Part model, mm, in its own coordinate system. A direction names the side the tool comes from. Give positions to 0.01 mm unless a question says otherwise; leave off trailing zeros. Order: outer loops, then holes, each group sorted by start corner. A loop starts at its lowest first (then second) coordinate and runs counter-clockwise, first axis right, second up.
1. Probe line 1 (X direction, y = 5, z = 11.25); line 2 (X direction, y = 24, z = 17); line 3 (Y direction, x = -4, z = 17.75). List the from-to ranges inside material, lowest first.
2. Drop flat-ended pins along their axis: pin 1 Ø2.5 at (x, y) = (-34.98, -1.92) entering from +Z; pin 2 Ø2 at (y, z) = (3.5, 11) entering from +X; pin 3 Ø3 at (x, z) = (2.5, 16) entering from -Y; pin 4 Ø3 at (y, z) = (-2, 14) entering from +X. Give the stop position or say it passes through.
3. Mould opens along X. For faces 1 (the flat face through (-1.737, 40.062, 13.944)), 2 (the flat face through (-37.48, 36, 11)), 3 (the flat face through (-38, 21, 18)) say: +X half, -X half, draft (parallel to the pull), parting line (faces both ways), or undercut.
4. Slice it at D-D on z = 16.5. List the corners of the cut face in (x, y).
5. Slice it at B-B on y = 19. List the corners of the cut face in (x, z).
6. Slice it at C-C on x = -10. List the corners of the cut face in (y, z).
7. Which spindle directions (+Z, -Z, +X, -X, +Y, -Y) get a long thin tool onto all of the face, cutting with end or side? Do faces 4 (the flat face through (-21, 42.38, 11)), 5 (the flat face through (-3.93, -2, 14)), 6 (the flat face through (-21, 2.38, 15)). Say none if no direction does.
Autodesk Inventor part; units mm, degrees
ref_plane "Work Plane1" through (0, 0, 10) normal (0, 0, 1) x (1, 0, 0)
ref_plane "YZ Plane" through (0, 0, 0) normal (1, 0, 0) x (0, 1, 0)
ref_plane "XZ Plane" through (0, 0, 0) normal (0, 1, 0) x (-1, 0, 0)
ref_plane "Work Plane1" through (0, 0, 10) normal (0, 0, 1) x (1, 0, 0)
sketch "Sketch1" plane through (0, 0, 10) normal (0, 0, 1) x (1, 0, 0)
  line L0 (-4.0299, -0.3538) -> (-2.2322, 1.4439) construction
  arc A0 (-1.4439, 2.2322) -> (-2.2322, 1.4439) centre (-0.9299, 0.9299) ccw construction
  line L1 (-1.4439, 2.2322) -> (0.3538, 4.0299) construction
  line L2 (-37.8299, 42.2137) -> (-37.8299, 45.8299) construction
  line L3 (-37.8299, 45.8299) -> (-4.0299, 45.8299) construction
  line L4 (-4.0299, 45.8299) -> (-4.0299, 42.2137) construction
  line L5 (-4.0299, 4.0299) -> (0.3538, 4.0299)
  circle A1 centre (-20.9299, 20.9299) radius 17.5 construction
  line L6 (-20.9299, 58.9723) -> (17.1124, 20.9299) construction
  line L7 (17.1124, 20.9299) -> (-20.9299, -17.1124) construction
  line L8 (-20.9299, -17.1124) -> (-58.9723, 20.9299) construction
  line L9 (-58.9723, 20.9299) -> (-20.9299, 58.9723) construction
  line L10 (-20.9299, 58.9723) -> (-20.9299, -17.1124) construction
  line L11 (17.1124, 20.9299) -> (-58.9723, 20.9299) construction
  line L12 (-20.9299, 58.9723) -> (32.8701, 58.9723) construction
  line L13 (-43.2198, 43.4299) -> (1.7802, 43.4299) construction
  line L14 (1.7802, 43.4299) -> (1.7802, -1.5701) construction
  line L15 (1.7802, -1.5701) -> (-43.2198, -1.5701) construction
  line L16 (-43.2198, -1.5701) -> (-43.2198, 43.4299) construction
  line L17 (-43.2198, 5.1774) -> (-43.2198, 36.6824)
  line L18 (-43.2198, 36.6824) -> (-36.4723, 43.4299)
  line L19 (-36.4723, 43.4299) -> (-5.3876, 43.4299)
  line L20 (-5.3876, 43.4299) -> (1.7802, 36.2621)
  line L21 (1.7802, 36.2621) -> (1.7802, 5.5977)
  line L22 (1.7802, 5.5977) -> (-5.3876, -1.5701)
  line L23 (-5.3876, -1.5701) -> (-36.4723, -1.5701)
  line L24 (-36.4723, -1.5701) -> (-43.2198, 5.1774)
  line L25 (-4.0299, 42.2137) -> (-37.8299, 42.2137)
  line L26 (-4.0299, -0.3538) -> (-4.0299, 4.0299)
  line L27 (-43.2198, 43.4299) -> (-10.4667, 10.6769) construction
  line L28 (-8.5595, 8.5517) -> (1.7802, -1.5701) construction
  line L29 (1.7802, 43.4299) -> (-25.699, 15.9507) construction
  line L30 (-30.9728, 10.6769) -> (-43.2198, -1.5701) construction
  point P0 (-37.8299, 4.0299)
  dimension "d18" = 53.8
  dimension "d19" = 45
  dimension "d20" = 53.8
  dimension "d21" = 45
  dimension "d22" = 45
extrude "Extrusion1" add sketch "Sketch1" along normal blind 8
sketch "Sketch3" plane through (0, 0, 10) normal (0, 0, -1) x (-1, 0, 0)
  line L0 (37.8299, -0.4701) -> (37.8299, 4.0299) construction
  line L1 (4.0299, 4.0299) -> (4.0299, -0.4701) construction
  line L2 (37.8299, -0.4701) -> (37.8299, 1.1886) construction
  line L3 (4.0299, -3.9701) -> (4.0299, -0.3538) construction
  line L4 (45.8299, 4.0299) -> (42.2137, 4.0299) construction
  line L5 (-0.3538, 4.0299) -> (-3.9701, 4.0299) construction
  line L6 (-3.9701, 37.8299) -> (-0.3538, 37.8299) construction
  line L7 (4.0299, 42.2137) -> (4.0299, 45.8299) construction
  line L8 (37.8299, 45.8299) -> (37.8299, 42.2137) construction
  line L9 (42.2137, 37.8299) -> (45.8299, 37.8299) construction
  line L10 (37.8299, 37.7299) -> (45.8299, 37.7299)
  line L11 (45.8299, 37.7299) -> (45.8299, 4.1299)
  line L12 (45.8299, 4.1299) -> (37.8299, 4.1299)
  line L13 (37.8299, 4.1299) -> (37.8299, 37.7299)
  line L14 (37.7299, 4.0299) -> (4.1299, 4.0299)
  line L15 (4.1299, 4.0299) -> (4.1299, -3.9701)
  line L16 (4.1299, -3.9701) -> (37.7299, -3.9701)
  line L17 (37.7299, -3.9701) -> (37.7299, 4.0299)
  line L18 (4.0299, 4.1299) -> (-3.9701, 4.1299)
  line L19 (-3.9701, 4.1299) -> (-3.9701, 37.7299)
  line L20 (-3.9701, 37.7299) -> (4.0299, 37.7299)
  line L21 (4.0299, 37.7299) -> (4.0299, 4.1299)
  line L22 (4.1299, 37.8299) -> (37.7299, 37.8299)
  line L23 (37.7299, 37.8299) -> (37.7299, 45.8299)
  line L24 (37.7299, 45.8299) -> (4.1299, 45.8299)
  line L25 (4.1299, 45.8299) -> (4.1299, 37.8299)
  point P0 (0, 0)
  dimension "d23" = 0.1
  dimension "d24" = 0.1
  dimension "d25" = 0.1
  dimension "d26" = 0.1
  dimension "d27" = 0.1
extrude "Extrusion3" add sketch "Sketch3" against normal up to surface (8 mm away)
sketch "Skizze12" plane through (0, 0, 10) normal (0, 0, -1) x (-1, 0, 0)
  line L0 (-0.3124, 4.1299) -> (4.1299, -0.3124)
  line L1 (4.1299, -0.3124) -> (4.1299, -3.9701)
  line L2 (4.1299, -3.9701) -> (37.7299, -3.9701) construction
  line L3 (37.7299, -3.9701) -> (37.7299, -0.3124)
  line L4 (37.7299, -0.3124) -> (42.1723, 4.1299)
  line L5 (45.8299, 4.1299) -> (42.1723, 4.1299)
  line L6 (45.8299, 37.7299) -> (45.8299, 4.1299) construction
  line L7 (42.1723, 37.7299) -> (45.8299, 37.7299)
  line L8 (42.1723, 37.7299) -> (37.7299, 42.1723)
  line L9 (37.7299, 42.1723) -> (37.7299, 45.8299)
  line L10 (37.7299, 45.8299) -> (4.1299, 45.8299) construction
  line L11 (4.1299, 45.8299) -> (4.1299, 42.1723)
  line L12 (4.1299, 42.1723) -> (-0.3124, 37.7299)
  line L13 (-3.9701, 37.7299) -> (-0.3124, 37.7299)
  line L14 (-3.9701, 4.1299) -> (-3.9701, 37.7299) construction
  line L15 (-0.3124, 4.1299) -> (-3.9701, 4.1299)
  line L16 (37.9299, -4.1701) -> (3.9299, -4.1701) construction
  line L17 (3.9299, -4.1701) -> (3.9299, -0.3953)
  line L18 (3.9299, -0.3953) -> (-0.3953, 3.9299)
  line L19 (-0.3953, 3.9299) -> (-4.1701, 3.9299)
  line L20 (-4.1701, 3.9299) -> (-4.1701, 37.9299) construction
  line L21 (-4.1701, 37.9299) -> (-0.3953, 37.9299)
  line L22 (-0.3953, 37.9299) -> (3.9299, 42.2551)
  line L23 (3.9299, 42.2551) -> (3.9299, 46.0299)
  line L24 (3.9299, 46.0299) -> (37.9299, 46.0299) construction
  line L25 (37.9299, 46.0299) -> (37.9299, 42.2551)
  line L26 (37.9299, 42.2551) -> (42.2551, 37.9299)
  line L27 (42.2551, 37.9299) -> (46.0299, 37.9299)
  line L28 (46.0299, 37.9299) -> (46.0299, 3.9299) construction
  line L29 (46.0299, 3.9299) -> (42.2551, 3.9299)
  line L30 (42.2551, 3.9299) -> (37.9299, -0.3953)
  line L31 (37.9299, -0.3953) -> (37.9299, -4.1701)
  line L32 (-3.9701, 37.7299) -> (-3.9701, 37.9299)
  line L33 (37.7299, 45.8299) -> (4.1299, 45.8299)
  line L34 (4.1299, 45.8299) -> (3.9299, 45.8299)
  line L35 (37.7299, 45.8299) -> (37.9299, 45.8299)
  line L36 (45.8299, 37.7299) -> (45.8299, 37.9299)
  line L37 (45.8299, 4.1299) -> (45.8299, 3.9299)
  line L38 (37.7299, -3.9701) -> (37.9299, -3.9701)
  line L39 (4.1299, -3.9701) -> (3.9299, -3.9701)
  line L40 (-3.9701, 4.1299) -> (-3.9701, 3.9299)
  point P0 (0, 0)
  dimension "d65" = 0.2
extrude "IM_offset" add sketch "Skizze12" against normal up to surface (8 mm away)
sketch "Sketch15" plane through (0, 0, 10) normal (0, 0, -1) x (-1, 0, 0)
  line L0 (-3.9701, 3.9299) -> (-3.9701, 37.9299)
  line L1 (-0.3953, 3.9299) -> (-3.9701, 3.9299)
  line L2 (3.9299, -0.3953) -> (-0.3953, 3.9299)
  line L3 (3.9299, -3.9701) -> (3.9299, -0.3953)
  line L4 (3.9299, -3.9701) -> (37.9299, -3.9701)
  line L5 (37.9299, -0.3953) -> (37.9299, -3.9701)
  line L6 (42.2551, 3.9299) -> (37.9299, -0.3953)
  line L7 (45.8299, 3.9299) -> (42.2551, 3.9299)
  line L8 (45.8299, 3.9299) -> (45.8299, 37.9299)
  line L9 (45.8299, 37.9299) -> (42.2551, 37.9299)
  line L10 (42.2551, 37.9299) -> (37.9299, 42.2551)
  line L11 (37.9299, 42.2551) -> (37.9299, 45.8299)
  line L12 (37.9299, 45.8299) -> (3.9299, 45.8299)
  line L13 (3.9299, 45.8299) -> (3.9299, 42.2551)
  line L14 (3.9299, 42.2551) -> (-0.3953, 37.9299)
  line L15 (-0.3953, 37.9299) -> (-3.9701, 37.9299)
  line L16 (37.4799, 42.3799) -> (4.4799, 42.3799)
  line L17 (4.4799, 42.3799) -> (4.4799, -0.6201)
  line L18 (4.4799, -0.6201) -> (37.4799, -0.6201)
  line L19 (37.4799, -0.6201) -> (37.4799, 42.3799)
  line L20 (37.4799, 42.3799) -> (4.4799, -0.6201) construction
  line L21 (4.4799, 42.3799) -> (37.4799, -0.6201) construction
  circle A0 centre (20.9799, 20.8799) radius 16.97 construction
  point P0 (0, 0)
  dimension "d73" = 33
  dimension "d74" = 43
  dimension "d90" = 21.5
  dimension "d91" = 16.5
extrude "Extrusion13" cut sketch "Sketch15" against normal blind 2 contours L19 L18 L17 L16
sketch "Sketch16" plane through (0, 0, 12) normal (0, 0, -1) x (-1, 0, 0)
  line L0 (4.4799, 42.3799) -> (37.4799, 42.3799)
  line L1 (4.4799, -0.6201) -> (4.4799, 42.3799)
  line L2 (37.4799, -0.6201) -> (4.4799, -0.6201)
  line L3 (37.4799, 42.3799) -> (37.4799, -0.6201)
  line L4 (7.4799, 39.3799) -> (34.4799, 39.3799)
  line L5 (34.4799, 39.3799) -> (34.4799, 2.3799)
  line L6 (34.4799, 2.3799) -> (7.4799, 2.3799)
  line L7 (7.4799, 2.3799) -> (7.4799, 39.3799)
  dimension "d94" = 3
extrude "Extrusion14" cut sketch "Sketch16" against normal through all contours L4 L5 L6 L7
sketch "Sketch17" plane through (0, 0, 10) normal (0, 0, -1) x (-1, 0, 0)
  line L0 (37.4799, 42.3799) -> (37.4799, -0.6201)
  line L1 (4.4799, -0.6201) -> (4.4799, 42.3799)
  line L2 (38.7299, 28.3799) -> (3.2299, 28.3799)
  line L3 (3.2299, 28.3799) -> (3.2299, 13.3799)
  line L4 (3.2299, 13.3799) -> (38.7299, 13.3799)
  line L5 (38.7299, 13.3799) -> (38.7299, 28.3799)
  line L6 (38.7299, 28.3799) -> (3.2299, 13.3799) construction
  line L7 (3.2299, 28.3799) -> (38.7299, 13.3799) construction
  line L8 (4.4799, 42.3799) -> (37.4799, 42.3799)
  circle A0 centre (20.9799, 20.8799) radius 16.97 construction
  line L9 (37.4799, -0.6201) -> (4.4799, -0.6201)
  point P0 (0, 0)
  dimension "d81" = 35.5
  dimension "d82" = 15
  dimension "d92" = 0
  dimension "d93" = 0
hole "Hole1" at (-3.2299, 13.3799, 10) at (-3.2299, 28.3799, 10) at (-38.7299, 28.3799, 10) at (-38.7299, 13.3799, 10) direction (0, 0, 1) diameter 2.8 end through all
sketch "Sketch18" plane through (0, 0, 10) normal (0, 0, -1) x (-1, 0, 0)
  line L0 (45.3299, 43.7299) -> (45.3299, -1.9701)
  line L1 (37.9499, -0.2701) -> (37.9499, -3.9701)
  line L2 (4.0099, -3.9701) -> (4.0099, 0.1299)
  circle A0 centre (6.9799, -1.9201) radius 1.4
  circle A1 centre (34.9799, -1.9201) radius 1.4
  circle A2 centre (20.9799, 20.8799) radius 16.97 construction
  circle A3 centre (20.9799, 20.8799) radius 16.97 construction
  point P0 (0, 0)
  dimension "d95" = 2.8
  dimension "d96" = 2.8
  dimension "d97" = 14
  dimension "d98" = 14
extrude "Extrusion15" cut sketch "Sketch18" against normal blind 10
properties part number "20_Cube_Insert_RaspiCam_v3"
Data:
1. line 1: x = -45.83 to -37.48, -4.48 to 3.97
1. line 2: x = -45.83 to -34.48, -7.48 to 3.97
1. line 3: y = -3.97 to 12.21, 14.55 to 27.21, 29.55 to 45.83
2. pin 1: passes through
2. pin 2: stops at x = 3.97
2. pin 3: stops at y = 3.93
2. pin 4: stops at x = -3.93
3. face 1: +X half
3. face 2: undercut
3. face 3: draft
4. outline: (-45.83, 3.93) - (-42.26, 3.93) - (-37.93, -0.4) - (-37.93, -3.97) - (-3.93, -3.97) - (-3.93, -0.4) - (0.4, 3.93) - (3.97, 3.93) - (3.97, 37.93) - (0.4, 37.93) - (-3.93, 42.26) - (-3.93, 45.83) - (-37.93, 45.83) - (-37.93, 42.26) - (-42.26, 37.93) - (-45.83, 37.93) - close; hole circle Ø2.8 at (-38.73, 13.38); hole circle Ø2.8 at (-38.73, 28.38); hole circle Ø2.8 at (-34.98, -1.92); hole (-34.48, 2.38) - (-7.48, 2.38) - (-7.48, 39.38) - (-34.48, 39.38) - close; hole circle Ø2.8 at (-6.98, -1.92); hole circle Ø2.8 at (-3.23, 13.38); hole circle Ø2.8 at (-3.23, 28.38)
5. outline: (-45.83, 10) - (-37.48, 10) - (-37.48, 12) - (-34.48, 12) - (-34.48, 18) - (-45.83, 18) - close; (-7.48, 12) - (-4.48, 12) - (-4.48, 10) - (3.97, 10) - (3.97, 18) - (-7.48, 18) - close
6. outline: (-3.97, 10) - (-0.62, 10) - (-0.62, 12) - (2.38, 12) - (2.38, 18) - (-3.97, 18) - close; (39.38, 12) - (42.38, 12) - (42.38, 10) - (45.83, 10) - (45.83, 18) - (39.38, 18) - close
7. face 4: -Z
7. face 5: +Z, -Z, +X, -Y
7. face 6: +Z, -Z
